Check sheet for the modelled part. Datum: model origin and axes. Units: mm. Round coordinates to 2 decimals unless told otherwise and drop trailing zeros. Write each loop counter-clockwise with the first axis right and the second up, starting at its lowest first coordinate (ties: lowest second). Pieces come first, ordered by that corner, then holes. Notation, with made-up numbers: (20, -16.75) -> (24, -16.75) arc R25 cw to (24, 15.25) -> close; hole circle Ø8 at (-36, 3). An arc over 180 degrees is marked (long way). Write item = value, one per line.
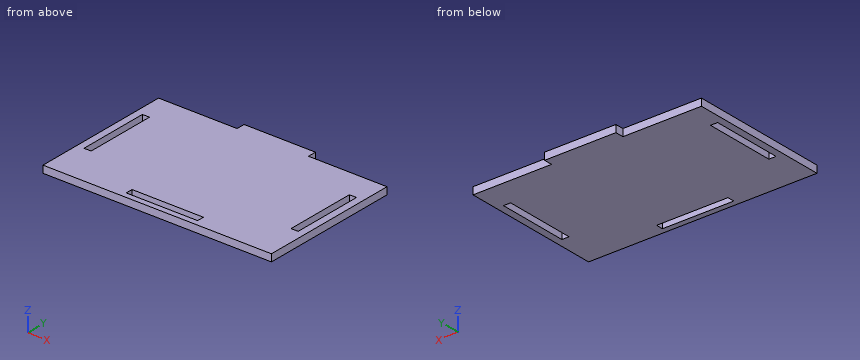
from build123d import *

# Parameters (mm, degrees)
SKETCH1_W           = 31.75
SKETCH1_H           = 3.175
SKETCH1_W_2         = 3.175
SKETCH1_H_2         = 31.75
BOSS_EXTRUDE1_DEPTH = 3.175


with BuildPart() as part:
    # Sketch1 → Boss-Extrude1 (new body)
    with BuildSketch(Plane.XY):
        Polygon((-50.8, 28.575), (-15.875, 28.575), (-15.875, 32.385), (15.875, 32.385), (15.875, 28.575), (50.8, 28.575), (50.8, -34.29), (-50.8, -34.29), align=None)
        with Locations((0, -30.1625)):
            Rectangle(SKETCH1_W, SKETCH1_H, mode=Mode.SUBTRACT)
        with Locations((-46.0375, 0)):
            Rectangle(SKETCH1_W_2, SKETCH1_H_2, mode=Mode.SUBTRACT)
        with Locations((46.0375, 0)):
            Rectangle(SKETCH1_W_2, SKETCH1_H_2, mode=Mode.SUBTRACT)
    extrude(amount=BOSS_EXTRUDE1_DEPTH)


solid = part.part
(1) Sectioned sample at C-C on z = 2.3. Enter the section's corners in (x, y) (3 decimals).
Worked answers:
outline = (-50.8, -34.29) -> (50.8, -34.29) -> (50.8, 28.575) -> (15.875, 28.575) -> (15.875, 32.385) -> (-15.875, 32.385) -> (-15.875, 28.575) -> (-50.8, 28.575) -> close; hole (-47.625, -15.875) -> (-44.45, -15.875) -> (-44.45, 15.875) -> (-47.625, 15.875) -> close; hole (-15.875, -31.75) -> (15.875, -31.75) -> (15.875, -28.575) -> (-15.875, -28.575) -> close; hole (44.45, -15.875) -> (47.625, -15.875) -> (47.625, 15.875) -> (44.45, 15.875) -> close
(2) Sectioned sample at D-D on x = 43. Enter the section's corners in (y, z) (3 decimals), then the cut area to 3 significant figures.
Worked answers:
outline = (-34.29, 0) -> (28.575, 0) -> (28.575, 3.175) -> (-34.29, 3.175) -> close
area = 200 mm²
(3) Go/stop test with flat-tipped pins: P1, Ø6, axis at x = 27, y = 13.5, coming from the -Z side; P2, Ø1, axis at y = 30, z = 1, coming from the +X side (3 decimals); P3, Ø1, axis at y = 31.5, z = 2, coming from the -X side (3 decimals); P4, Ø1.6, axis at x = -45.5, z = 1.5, coming from the +Y side (3 decimals). Record where each tip stops, or that it passes through.
Worked answers:
P1 = 0
P2 = 15.875
P3 = -15.875
P4 = 28.575
(4) Sectioned sample at A-A on x = -12.5. Enter the section's corners in (y, z) (3 decimals), then the cut area to 3 significant figures.
Worked answers:
outline = (-34.29, 0) -> (-31.75, 0) -> (-31.75, 3.175) -> (-34.29, 3.175) -> close; (-28.575, 0) -> (32.385, 0) -> (32.385, 3.175) -> (-28.575, 3.175) -> close
area = 202 mm²
(5) Sectioned sample at B-B on y = 12.5. Enter the section's corners in (x, z) (3 decimals).
Worked answers:
outline = (-50.8, 0) -> (-47.625, 0) -> (-47.625, 3.175) -> (-50.8, 3.175) -> close; (-44.45, 0) -> (44.45, 0) -> (44.45, 3.175) -> (-44.45, 3.175) -> close; (47.625, 0) -> (50.8, 0) -> (50.8, 3.175) -> (47.625, 3.175) -> close
(6) Material ranges on L1, parallel to X at y = 4, z = 1.8 (3 decimals); L2, parallel to Y at x = -4.5, z = 0.85 (3 decimals); L3, parallel to Y at x = -17, z = 0.25 (3 decimals), recorded low to high. Write a range as [from, to].
Worked answers:
L1 = [-50.8, -47.625], [-44.45, 44.45], [47.625, 50.8]
L2 = [-34.29, -31.75], [-28.575, 32.385]
L3 = [-34.29, 28.575]
